Autodesk Fusion 360 part; units mm, degrees
sketch "Sketch1" plane through (0, 0, 0) normal (0, 0, 1) x (1, 0, 0)
  line L0 (0, 13) -> (44.5, 13)
  line L1 (0, 0) -> (-1, 0)
  line L2 (-1, 0) -> (-1, 6)
  line L3 (-1, 6) -> (0, 6)
  line L4 (0, -9) -> (27.5027, -9)
  line L5 (44.5, 13) -> (44.5, -4.4456)
  line L6 (9.2672, -6.9165) -> (19.8794, -6.9165) construction
  line L7 (25.7993, -4.4556) -> (22.983, 6.4362)
  line L8 (22.983, 6.4362) -> (39.6837, 10.7545)
  line L9 (39.6837, 10.7545) -> (42.5, -0.1373)
  line L10 (0, 13) -> (0, 6)
  line L11 (0, 0) -> (0, -9)
  line L12 (27.5027, -9) -> (28.2069, -8.8113)
  line L13 (27.5027, -9) -> (27.6263, -9) construction
  line L14 (28.5868, -5.749) -> (28.0986, -3.8611)
  line L15 (40.6888, -2.6198) -> (40.2006, -0.7319)
  line L16 (28.0986, -3.8611) -> (25.7993, -4.4556)
  line L17 (40.2006, -0.7319) -> (42.5, -0.1373)
  line L18 (28.5868, -5.749) -> (40.6888, -2.6198)
  line L19 (28.2069, -8.8113) -> (44.5, -4.4456)
  point P0 (28.5868, -5.749)
  dimension "d1" = 44.5
  dimension "d3" = 1
  dimension "d4" = 6
  dimension "d6" = 9
  dimension "d7" = 7
  dimension "d15" = 17.25
  dimension "d25" = 15
  dimension "d26" = 12.5
  dimension "d30" = 2
  dimension "d31" = 105
  dimension "d33" = 2.75
  dimension "d34" = 13.2
  dimension "d35" = 16.9973
  dimension "d38" = 11.25
extrude "Extrude1" add sketch "Sketch1" along normal blind 10
sketch "Sketch2" plane through (-1, 0, 0) normal (-1, 0, 0) x (0, 0, 1)
  line L0 (0, 6) -> (0, 0)
  line L1 (0, 0) -> (10, 0)
  line L2 (10, 0) -> (10, 6)
  line L3 (10, 6) -> (0, 6)
  circle A0 centre (5, 3) radius 1.6
  circle A1 centre (5, 3) radius 3
  dimension "d18" = 3.2
  dimension "d19" = 6
extrude "Extrude2" cut sketch "Sketch2" against normal up to surface (45.5 mm away) contours A0
ref_plane "WorkPlane1" through (26, 3, 5) normal (-1, 0, 0) x (0, 0, 1)
sketch "Sketch3" plane through (26, 3, 2.5) normal (-1, 0, 0) x (0, 0, -1)
  circle A0 centre (-2.5, 0) radius 3
  point P0 (-2.5, 0)
extrude "Extrude3" cut sketch "Sketch3" along normal blind 23
equation "d1 = 27.5 mm + 17 mm"
equation "d23 = 27 mm - 4 mm"
The listing builds one solid part. Answer for the finished solid, in the listing's coordinates (mm). A direction names the side the tool comes from. Round coordinates to 2 decimals unless told otherwise and drop trailing zeros. Order: outer loops, then holes, each group sorted by start corner. A loop starts at its lowest first (then second) coordinate and runs counter-clockwise, first axis right, second up. Notation, with made-up numbers: (15, 52) -> (58, 52) arc R21 ccw to (58, 86) -> close; hole circle Ø11 at (77, -39.5). An arc over 180 degrees is marked (long way). Put each result on its own line as item: value.
Q1. Section B-B, the plane z = 9.25 is taken. Write down the section's boundary in (x, y), and give its area (3 significant figures).
Results list:
outline: (-1, 0) -> (0, 0) -> (0, -9) -> (27.5, -9) -> (28.21, -8.81) -> (44.5, -4.45) -> (44.5, 13) -> (0, 13) -> (0, 6) -> (-1, 6) -> close; hole (22.98, 6.44) -> (25.8, -4.46) -> (28.1, -3.86) -> (28.59, -5.75) -> (40.69, -2.62) -> (40.2, -0.73) -> (42.5, -0.14) -> (39.68, 10.75) -> close
area: 728 mm^2
Q2. Consider line 1 along Y through (x, z) = (6, 5); line 2 along Z through (x, y) = (11, 3); line 3 along Z through (x, y) = (43.75, 3). Determine where each line is inside the solid, lowest interval first.
Results list:
line 1: -9 to 0, 6 to 13
line 2: 0 to 2, 8 to 10
line 3: 0 to 3.4, 6.6 to 10
Q3. Determine the mould class of faces 4 (the flat face through (3, 4.3, 3.7)), 5 (the flat face through (0, 10, 5)), 6 (the flat face through (-0.5, 6, 4.9)), 7 (the flat face through (31.216, 8.565, 4.93)) for opening direction X: pulls with the +X half, pulls with the -X half, needs draft (parallel to the pull), parting line crosses it, or undercut.
Results list:
face 4: undercut
face 5: pulls with the -X half
face 6: needs draft
face 7: undercut
Q4. Section A-A, the plane y = 9.5 is taken. Write down the section's boundary in (x, z).
Results list:
outline: (0, 0) -> (34.83, 0) -> (34.83, 10) -> (0, 10) -> close; (40.01, 0) -> (44.5, 0) -> (44.5, 10) -> (40.01, 10) -> close
Q5. Which of the six approach directions +Z, -Z, +X, -X, +Y, -Y give full straight-line access (tool end or side, diameter ignored) to faces 1 (the flat face through (24.724, -0.296, 4.93)), 2 (the cylindrical face through (13.976, 0.338, 3.616)), 3 (the flat face through (0, -4, 5))?
Results list:
face 1: +Z, -Z
face 2: none
face 3: +Z, -Z, -X, -Y
Q6. Each of these flat-tipped pins is pushed along its axis until it touches: P1, Ø0.8, axis at x = -0.5, z = 7.5, coming from the +Y side; P2, Ø3, axis at y = -7, z = 4.5, coming from the -X side; P3, Ø0.8, axis at x = -0.5, z = 5, coming from the -Y side; P4, Ø4, axis at x = 13.5, y = -3.5, coming from the -Z side. Where does it stop, or does it pass through?
Results list:
P1: y = 6
P2: x = 0
P3: y = 0
P4: z = 0
Q7. Section D-D, the plane y = 3 is taken. Write down the section's boundary in (x, z), and give its area (3 significant figures).
Results list:
outline: (-1, 0) -> (23.87, 0) -> (23.87, 2) -> (3, 2) -> (3, 3.4) -> (-1, 3.4) -> close; (-1, 6.6) -> (3, 6.6) -> (3, 8) -> (23.87, 8) -> (23.87, 10) -> (-1, 10) -> close; (41.69, 0) -> (44.5, 0) -> (44.5, 3.4) -> (41.69, 3.4) -> close; (41.69, 6.6) -> (44.5, 6.6) -> (44.5, 10) -> (41.69, 10) -> close
area: 130 mm^2
